```python
from build123d import *

# Parameters (mm, degrees)
F0_W     = 50
F0_H     = 17.6952143589
F1_DEPTH = 5
F2_D     = 6
F2_DEPTH = 12
F2_TIP   = 1.8025818571
F3_D     = 5.9
F3_DEPTH = 12
F3_TIP   = 1.7725388261
F4_D     = 5.8
F4_DEPTH = 12
F4_TIP   = 1.7424957952
F5_D     = 5.7
F5_DEPTH = 12
F5_TIP   = 1.7124527642
F6_D     = 5.6
F6_DEPTH = 12
F6_TIP   = 1.6824097333
F7_D     = 5.5
F7_DEPTH = 12
F7_TIP   = 1.6523667023


with BuildPart() as f1:
    # F0 (on Top) → F1 (new body)
    with BuildSketch(Plane.XY):
        with Locations((0.0939741731, -0.1879474148)):
            Rectangle(F0_W, F0_H)
    extrude(amount=F1_DEPTH)

    # F2
    with Locations(Plane(origin=(0, 0, 0), x_dir=(1, 0, 0), z_dir=(0, 0, -1))):
        with Locations((-15.8815626055, -2.5372912642)):
            Hole(F2_D / 2, depth=F2_DEPTH)
            with Locations((0, 0, -(F2_DEPTH + F2_TIP / 2))):  # 118° drill point
                Cone(0, F2_D / 2, F2_TIP, mode=Mode.SUBTRACT)

    # F3
    with Locations(Plane(origin=(0, 0, 0), x_dir=(1, 0, 0), z_dir=(0, 0, -1))):
        with Locations((-8.0951671781, -2.5372912642)):
            Hole(F3_D / 2, depth=F3_DEPTH)
            with Locations((0, 0, -(F3_DEPTH + F3_TIP / 2))):  # 118° drill point
                Cone(0, F3_D / 2, F3_TIP, mode=Mode.SUBTRACT)

    # F4
    with Locations(Plane(origin=(0, 0, 0), x_dir=(1, 0, 0), z_dir=(0, 0, -1))):
        with Locations((-1.7855006403, -2.5372912642)):
            Hole(F4_D / 2, depth=F4_DEPTH)
            with Locations((0, 0, -(F4_DEPTH + F4_TIP / 2))):  # 118° drill point
                Cone(0, F4_D / 2, F4_TIP, mode=Mode.SUBTRACT)

    # F5
    with Locations(Plane(origin=(0, 0, 0), x_dir=(1, 0, 0), z_dir=(0, 0, -1))):
        with Locations((5.5981517902, -2.5372912642)):
            Hole(F5_D / 2, depth=F5_DEPTH)
            with Locations((0, 0, -(F5_DEPTH + F5_TIP / 2))):  # 118° drill point
                Cone(0, F5_D / 2, F5_TIP, mode=Mode.SUBTRACT)

    # F6
    with Locations(Plane(origin=(0, 0, 0), x_dir=(1, 0, 0), z_dir=(0, 0, -1))):
        with Locations((12.3105607927, -2.5372912642)):
            Hole(F6_D / 2, depth=F6_DEPTH)
            with Locations((0, 0, -(F6_DEPTH + F6_TIP / 2))):  # 118° drill point
                Cone(0, F6_D / 2, F6_TIP, mode=Mode.SUBTRACT)

    # F7
    with Locations(Plane(origin=(0, 0, 0), x_dir=(1, 0, 0), z_dir=(0, 0, -1))):
        with Locations((20.2312065022, -2.5372912642)):
            Hole(F7_D / 2, depth=F7_DEPTH)
            with Locations((0, 0, -(F7_DEPTH + F7_TIP / 2))):  # 118° drill point
                Cone(0, F7_D / 2, F7_TIP, mode=Mode.SUBTRACT)


solid = f1.part
```
Work out the finished part from the listing and answer in its coordinate system (mm). Coordinates: 2 decimals unless noted, no trailing zeros. Loops run counter-clockwise (first coordinate to the right, second up) from the corner with the lowest first, then second, coordinate; pieces in that order, holes last. Notation, with made-up numbers: M -3,17.25 L 40,17.25 A18 cw 40,21.25 Z; hole C 5,22 d7. An arc over 180 degrees is marked long. Use CSV: the item, a comma, the result in double quotes. Start each with the question number.
(1) Consider line 1 (Y direction, x = 10, z = 1.6); line 2 (Y direction, x = -3.5, z = 4.3). Determine where each line is inside the solid, lowest interval first.
(2) For a pull along X with two mould halves and no side action, classify faces 1 (the face through (0, 0, 5)), 2 (the face through (25.094, 0, 2)), 3 (the face through (-3.34, 0.09, 2.54)) as +X half, -X half, draft (parallel to the pull), parting line (faces both ways), or undercut.
(3) Find section C-C, the plane z = 2.45. Give the vertices of the cut face in (x, y).
(4) Find section D-D, the plane y = 4. Give the vertices of the cut face in (x, z), then the cut area to 3 significant figures.
(5) Find section B-B, the plane x = -3. Give the vertices of the cut face in (y, z), then the cut area to 3 significant figures.
(6) Find section A-A, the plane y = 1. Give the vertices of the cut face in (x, z), then the cut area to 3 significant figures.
Recorded:
1,line 1,"y = -9.04 to 0.96, 4.12 to 8.66"
1,line 2,"y = -9.04 to 0.2, 4.88 to 8.66"
2,face 1,"draft"
2,face 2,"+X half"
2,face 3,"undercut"
3,outline,"M -24.91,-9.04 L 25.09,-9.04 L 25.09,8.66 L -24.91,8.66 Z; hole C -15.88,2.54 d6; hole C -8.1,2.54 d5.9; hole C -1.79,2.54 d5.8; hole C 5.6,2.54 d5.7; hole C 12.31,2.54 d5.6; hole C 20.23,2.54 d5.5"
4,outline,"M -24.91,0 L -18.5,0 L -18.5,5 L -24.91,5 Z; M -13.26,0 L -10.66,0 L -10.66,5 L -13.26,5 Z; M -5.53,0 L -4.29,0 L -4.29,5 L -5.53,5 Z; M 0.72,0 L 3.15,0 L 3.15,5 L 0.72,5 Z; M 8.04,0 L 9.92,0 L 9.92,5 L 8.04,5 Z; M 14.7,0 L 17.9,0 L 17.9,5 L 14.7,5 Z; M 22.56,0 L 25.09,0 L 25.09,5 L 22.56,5 Z"
4,area,"102 mm^2"
5,outline,"M -9.04,0 L -0.1,0 L -0.1,5 L -9.04,5 Z; M 5.17,0 L 8.66,0 L 8.66,5 L 5.17,5 Z"
5,area,"62.1 mm^2"
6,outline,"M -24.91,0 L -18.46,0 L -18.46,5 L -24.91,5 Z; M -13.31,0 L -10.61,0 L -10.61,5 L -13.31,5 Z; M -5.58,0 L -4.24,0 L -4.24,5 L -5.58,5 Z; M 0.67,0 L 3.2,0 L 3.2,5 L 0.67,5 Z; M 8,0 L 9.97,0 L 9.97,5 L 8,5 Z; M 14.65,0 L 17.95,0 L 17.95,5 L 14.65,5 Z; M 22.51,0 L 25.09,0 L 25.09,5 L 22.51,5 Z"
6,area,"104 mm^2"
